from build123d import *

# Parameters (mm, degrees)
F0_W     = 38.2413167982
F0_H     = 130.5519748793
F1_DEPTH = 19.05


with BuildPart() as f1:
    # F0 (on Front) → F1 (new body)
    with BuildSketch(Plane.XZ):
        with Locations((-5e-10, 64.9347287138)):
            Rectangle(F0_W, F0_H)
        with BuildLine():
            Line((-19.1206583996, 130.2107161535), (19.1206583986, 130.2107161535))
            Line((19.1206583986, 130.2107161535), (25.4706583986, 130.2107161535))
            add(Edge.make_bspline(
                [(25.4706583986, 130.2107161535), (30.0724719756, 169.0966659039), (51.3980125218, 257.0949252577), (168.2834825455, 304.8190286771), (326.925094009, 369.4938490194), (396.8974330576, 452.268946401), (393.7810574923, 535.008276766), (377.0494931199, 592.3264271799), (368.2999999833, 622.3000000618)],
                knots=[0.1131891299, 0.1131891299, 0.1131891299, 0.1131891299, 0.2225944071, 0.3940346608, 0.5865569639, 0.732236582, 0.8599775765, 1, 1, 1, 1], degree=3))
            ThreePointArc((368.2999999833, 622.3000000618), (-1.67e-08, 681.4277668685), (-368.3000000167, 622.3000000618))
            add(Edge.make_bspline(
                [(-25.4706584275, 130.2107161535), (-30.0724720137, 169.0966658909), (-51.3980125817, 257.094925206), (-168.2834825322, 304.8190286898), (-326.9250939954, 369.4938490451), (-396.8974330089, 452.2689464188), (-393.781057464, 535.008276759), (-377.0494931536, 592.3264271786), (-368.3000000167, 622.3000000618)],
                knots=[0.1131891299, 0.1131891299, 0.1131891299, 0.1131891299, 0.222594407, 0.3940346608, 0.5865569639, 0.7322365819, 0.8599775765, 1, 1, 1, 1], degree=3))
            Line((-25.4706584275, 130.2107161535), (-19.1206583996, 130.2107161535))
        make_face()
    extrude(amount=F1_DEPTH)


solid = f1.part
Geometry: final body of the model. Coordinates: model frame, mm. A direction names the side the tool comes from. Give positions to 0.01 mm unless a question says otherwise; leave off trailing zeros. Put each result on its own line as item: value.
1) Material intervals for L1, parallel to X at y = -3.25, z = 49; L2, parallel to Z at x = -4, y = -5; L3, parallel to Z at x = 349.5, y = -5.5, sorted ascending. Write a range as from..to.
Computed values:
L1: x = -19.12..19.12
L2: z = -0.34..681.42
L3: z = 401.91..628.32
2) Reachability of faces 1 (the flat face through (-19.121, -9, 64)), 2 (the flat face through (-6, 0, 497)) from +Z, -Z, +X, -X, +Y, -Y: full face, straight path, thin tool, end or side. Return the list, or none.
Computed values:
face 1: -Z, -X, +Y, -Y
face 2: +Z, -Z, +X, -X, +Y
3) Mould query, pull axis Z, two halves, no side actions, for faces 3 (the flat face through (19.121, -9, 64)), 4 (the cylindrical face through (5.244, -9.392, 681.416)), 5 (the flat face through (0, -9, -0.341)). Classes: released by +Z, released by -Z, zero draft, split by the parting line, or undercut.
Computed values:
face 3: zero draft
face 4: released by +Z
face 5: released by -Z
4) First-contact query: P1, Ø3, axis at y = -17, z = 352.5, coming from the +X side; P2, Ø3, axis at x = 250.5, z = 415, coming from the +Y side; P3, Ø10, axis at y = -12, z = 338, coming from the +X side; P4, Ø5.5, axis at y = -11, z = 97.5, coming from the -X side. Flat tips, straight axial feed; report the tip coordinate or a pass-through.
Computed values:
P1: stops at x = 278.98
P2: stops at y = 0
P3: stops at x = 256.96
P4: stops at x = -19.12
